```python
from build123d import *


with BuildPart() as part:
    # Sketch1 → Revolve-Thin1 (revolve)
    with BuildSketch(Plane.XY):
        with BuildLine():
            Line((5, 0), (11.22679428, 0))
            ThreePointArc((11.22679428, 0), (12.84785708, -0.343204217), (14.190742085, -1.313922301))
            Line((14.190742085, -1.313922301), (40.809257915, -30.686077699))
            ThreePointArc((40.809257915, -30.686077699), (42.15214292, -31.656795783), (43.77320572, -32))
            Line((43.77320572, -32), (46, -32))
            Line((46, -32), (46, -31))
            Line((46, -31), (43.77320572, -31))
            ThreePointArc((43.77320572, -31), (42.55740862, -30.742596837), (41.550244866, -30.014558274))
            Line((41.550244866, -30.014558274), (14.931729037, -0.642402876))
            ThreePointArc((14.931729037, -0.642402876), (13.25312278, 0.570994729), (11.22679428, 1))
            Line((11.22679428, 1), (5, 1))
            Line((5, 1), (5, 0))
        make_face()
    revolve(axis=Axis((0, 23.415841584, 0), (0, -1, 0)))


solid = part.part
```
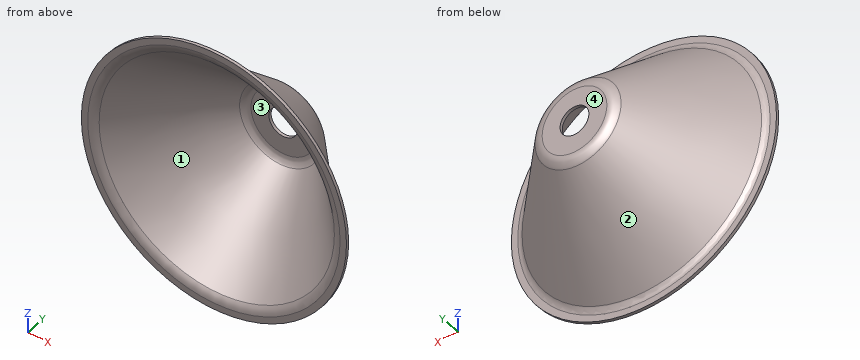
Check sheet for the modelled part. Datum: model origin and axes. Units: mm. Face numbers are marked on the shaded views. Round coordinates to 2 decimals unless told otherwise and drop trailing zeros. Order: outer loops, then holes, each group sorted by start corner. A loop starts at its lowest first (then second) coordinate and runs counter-clockwise, first axis right, second up. Notation, with made-up numbers: (-34, -38) - (-2, -38) arc R30 ccw to (-2, -11) - close; hole circle Ø10 at (-21.75, 67.5). An arc over 180 degrees is marked (long way). Answer as CSV lines item,"result". Start each with the question number.
1) Section check C-C (y = -12). Record the cut outline in (x, z) (3 decimals), then the cut area to 3 significant figures.
2) Section check D-D (y = -25). Record the cut outline in (x, z), then the cut area to 3 significant figures.
3) Section check B-B (x = 0). Record the cut outline in (y, z), then the cut area to 3 significant figures.
4) Draft check along X on the marked faces 1, 2, 3 and 4. Enter one of: +X half, -X half, draft (parallel to the pull), parting line (faces both ways), or undercut.
5) Depth check by flat-ended pin: pin 1 (5 mm diameter, centred on x = 15, y = -3, fed in from -Z); pin 2 (11 mm diameter, centred on x = 5, z = 0.5, fed in from -Y); pin 3 (1.5 mm diameter, centred on x = -6, z = -30, fed in from -Y). Enter the tip coordinate at first touch or a pass-through.
6) Section check A-A (z = 0). Record the cut outline in (x, y), then the cut area to 3 significant figures.
7) Scan lines: probe 1 along Y at (x, z) = (-15, 41); probe 2 along X at (y, z) = (-4, -0.5); probe 3 along X at (y, z) = (-21.5, 29). Record each from-to range of solid material in increasing order.
Determined:
1,outline,"circle Ø50.449 at (0, 0); hole circle Ø47.75 at (0, 0)"
1,area,"208 mm^2"
2,outline,"circle Ø74.01 at (0, 0); hole circle Ø71.31 at (0, 0)"
2,area,"308 mm^2"
3,outline,"(-32, -46) - (-31, -46) - (-31, -43.77) arc R3 cw to (-30.01, -41.55) - (-0.64, -14.93) arc R5 ccw to (1, -11.23) - (1, -5) - (0, -5) - (0, -11.23) arc R4 cw to (-1.31, -14.19) - (-30.69, -40.81) arc R4 ccw to (-32, -43.77) - close; (-32, 43.77) arc R4 ccw to (-30.69, 40.81) - (-1.31, 14.19) arc R4 cw to (0, 11.23) - (0, 5) - (1, 5) - (1, 11.23) arc R5 ccw to (-0.64, 14.93) - (-30.01, 41.55) arc R3 cw to (-31, 43.77) - (-31, 46) - (-32, 46) - close"
3,area,"110 mm^2"
4,face 1,"undercut"
4,face 2,"parting line"
4,face 3,"undercut"
4,face 4,"draft"
5,pin 1,"z = -13.2"
5,pin 2,"y = 0"
5,pin 3,"y = -20.24"
6,outline,"(-46, -32) - (-43.77, -32) arc R4 ccw to (-40.81, -30.69) - (-14.19, -1.31) arc R4 cw to (-11.23, 0) - (-5, 0) - (-5, 1) - (-11.23, 1) arc R5 ccw to (-14.93, -0.64) - (-41.55, -30.01) arc R3 cw to (-43.77, -31) - (-46, -31) - close; (5, 0) - (11.23, 0) arc R4 cw to (14.19, -1.31) - (40.81, -30.69) arc R4 ccw to (43.77, -32) - (46, -32) - (46, -31) - (43.77, -31) arc R3 cw to (41.55, -30.01) - (14.93, -0.64) arc R5 ccw to (11.23, 1) - (5, 1) - close"
6,area,"110 mm^2"
7,probe 1,"-32 to -31"
7,probe 2,"-17.97 to -16.62, 16.62 to 17.97"
7,probe 3,"-17.43 to -14.64, 14.64 to 17.43"
